Check sheet for the modelled part. Datum: model origin and axes. Units: mm. Face numbers are marked on the shaded views. A direction names the side the tool comes from. Give positions to 0.01 mm unless a question says otherwise; leave off trailing zeros. Loops run counter-clockwise (first coordinate to the right, second up) from the corner with the lowest first, then second, coordinate; pieces in that order, holes last. Notation, with made-up numbers: M 50.25,-2 L 71.25,-2 A33 ccw 71.25,30 Z; hole C 4,68 d11. An arc over 180 degrees is marked long. Write each question's results on one line, items separated by ' | '. Start each with the question number.
1. Sectioned sample at C-C on z = -3. Record the cut outline in (x, y), and give its area (3 significant figures).
2. Go/stop test with flat-tipped pins: pin 1 (7 mm diameter, centred on x = 32, y = 21.5, fed in from -Z); pin 2 (3 mm diameter, centred on y = 42.5, z = -22, fed in from +X); pin 3 (10.5 mm diameter, centred on x = -37, z = 9.5, fed in from -Y). Record where each tip stops, or that it passes through.
3. Sectioned sample at D-D on x = -39. Record the cut outline in (y, z), and give its area (3 significant figures).
4. Tool access check on the marked faces 5 and 6. Record the directions out of +Z, -Z, +X, -X, +Y, -Y that give a thin tool (end or side, any length) a straight path to the whole face; none if there is none.
5. Sectioned sample at B-B on y = 29. Record the cut outline in (x, z).
6. Material ranges on line 1 along Z through (x, y) = (0, 35); line 2 along X through (y, z) = (32, 0); line 3 along Z through (x, y) = (21, 21), recorded low to high.
7. Sectioned sample at A-A on x = 0. Record the cut outline in (y, z).
8. Draft check along Y on the marked faces 1, 2, 3 and 4. Enter one of: pulls with the +Y half, pulls with the -Y half, needs draft (parallel to the pull), parting line crosses it, or undercut.
```python
from build123d import *

# Parameters (mm, degrees)
SKETCH1_R           = 50.8
BOSS_EXTRUDE1_DEPTH = 50.8
SKETCH2_W           = 101.6
SKETCH2_H           = 101.6
CUT_EXTRUDE1_DEPTH  = 50.8
SKETCH3_W           = 101.6
SKETCH3_H           = 50.8
BOSS_EXTRUDE2_DEPTH = 25.4
SKETCH4_R           = 19.150000054
CUT_EXTRUDE2_DEPTH  = 50.8
CAVITY1_START       = -50.8
CAVITY1_DEPTH       = 101.6
SKETCH7_W           = 101.6
SKETCH7_H           = 22.400006
CUT_EXTRUDE3_DEPTH  = 0.2
SKETCH8_W           = 101.6
SKETCH8_H           = 4.242632202
CUT_EXTRUDE4_DEPTH  = 0.2
SKETCH9_W           = 101.6
SKETCH9_H           = 12.9
CUT_EXTRUDE5_DEPTH  = 0.2
SKETCH12_W          = 101.6
SKETCH12_H          = 6.55
CUT_EXTRUDE8_DEPTH  = 0.2
SKETCH13_W          = 101.6
SKETCH13_H          = 7.332348419
CUT_EXTRUDE9_DEPTH  = 0.2
FILLET3_R           = 0.2
FILLET4_R           = 0.2


with BuildPart() as part:
    # Sketch1 → Boss-Extrude1 (new body)
    with BuildSketch(Plane(origin=(0, 0, 0), x_dir=(1, 0, 0), z_dir=(0, 1, 0))):
        with Locations(Location((0, 0, 0), (0, 0, 270))):
            Circle(SKETCH1_R)
    extrude(amount=BOSS_EXTRUDE1_DEPTH)

    # Sketch2 → Cut-Extrude1 (cut)
    with BuildSketch(Plane(origin=(0, 50.8, 0), x_dir=(1, 0, 0), z_dir=(0, 1, 0))):
        with Locations((0, -50.8)):
            Rectangle(SKETCH2_W, SKETCH2_H)
    extrude(amount=-CUT_EXTRUDE1_DEPTH, mode=Mode.SUBTRACT)

    # Sketch3 → Boss-Extrude2 (add)
    with BuildSketch(Plane.XY):
        with Locations((0, 25.4)):
            Rectangle(SKETCH3_W, SKETCH3_H)
    extrude(amount=BOSS_EXTRUDE2_DEPTH)

    # Sketch4 → Cut-Extrude2 (cut)
    with BuildSketch(Plane(origin=(0, 50.8, 0), x_dir=(1, 0, 0), z_dir=(0, 1, 0))):
        with Locations(Location((0, 0, 0), (0, 0, 270))):
            Circle(SKETCH4_R)
    extrude(amount=-CUT_EXTRUDE2_DEPTH, mode=Mode.SUBTRACT)

    # Cavity1: read off the stored shape, not the designer's step
    # Cavity1 outline → Cavity1 (cut)
    with BuildSketch(Plane.YZ.offset(CAVITY1_START)):
        Polygon((19.05, 12.9), (12.7, 9.233825791), (12.7, 25.4), (0, 25.4), (0, 3.199994), (2.999994, 0.2), (25.4, 0.2), (25.4, 12.9), align=None)
    extrude(amount=CAVITY1_DEPTH, mode=Mode.SUBTRACT)

    # Sketch7 → Cut-Extrude3 (cut)
    with BuildSketch(Plane.XY.offset(0.2)):
        with Locations((0, 14.199997)):
            Rectangle(SKETCH7_W, SKETCH7_H)
    extrude(amount=-CUT_EXTRUDE3_DEPTH, mode=Mode.SUBTRACT)

    # Sketch8 → Cut-Extrude4 (cut)
    with BuildSketch(Plane(origin=(0, 1.599997, 1.599997), x_dir=(1, 0, 0), z_dir=(0, 0.7071067811865475, 0.7071067811865477))):
        with Locations((0, -0.141421356)):
            Rectangle(SKETCH8_W, SKETCH8_H)
    extrude(amount=-CUT_EXTRUDE4_DEPTH, mode=Mode.SUBTRACT)

    # Sketch9 → Cut-Extrude5 (cut)
    with BuildSketch(Plane.XZ.offset(-25.4)):
        with Locations((0, 6.45)):
            Rectangle(SKETCH9_W, SKETCH9_H)
    extrude(amount=-CUT_EXTRUDE5_DEPTH, mode=Mode.SUBTRACT)

    # Sketch12 → Cut-Extrude8 (cut)
    with BuildSketch(Plane(origin=(0, 0, 12.9), x_dir=(-1, 0, 0), z_dir=(0, 0, -1))):
        with Locations((0, 22.325)):
            Rectangle(SKETCH12_W, SKETCH12_H)
    extrude(amount=-CUT_EXTRUDE8_DEPTH, mode=Mode.SUBTRACT)

    # Sketch13 → Cut-Extrude9 (cut)
    with BuildSketch(Plane(origin=(0, -0.823363854, 1.426108029), x_dir=(-1, 0, 0), z_dir=(0, 0.4999999999999968, -0.8660254037844406))):
        with Locations((0, 19.281609733)):
            Rectangle(SKETCH13_W, SKETCH13_H)
    extrude(amount=-CUT_EXTRUDE9_DEPTH, mode=Mode.SUBTRACT)

    # Fillet3
    # the kernel refuses this fillet: 0.2 mm, written as the material it takes off along each edge
    with BuildSketch(Plane(origin=(-51.3, 19.05, 12.9), x_dir=(0, -1.0658141036380147e-12, 1.0), z_dir=(1, 0, 0))) as fillet3_piece_1:
        with BuildLine():
            CenterArc((0.373205081, 0.1), FILLET3_R, 180, 30)
            Line((0.173205081, 0.1), (0, 0))
            Line((0, 0), (0.2, 0))
        make_face()
    extrude(amount=37.646820072, mode=Mode.SUBTRACT)
    with BuildSketch(Plane(origin=(13.653179928, 19.05, 12.9), x_dir=(0, -0.4999999999991145, 0.86602540378495), z_dir=(1, 0, 0))) as fillet3_piece_2:
        with BuildLine():
            CenterArc((0.373205081, -0.1), FILLET3_R, 150, 30)
            Line((0.173205081, -0.1), (0, 0))
            Line((0, 0), (0.2, 0))
        make_face()
    extrude(amount=37.646820072, mode=Mode.SUBTRACT)

    # Fillet4
    # the kernel refuses this fillet: 0.2 mm, written as the material it takes off along each edge
    with BuildSketch(Plane(origin=(-51.3, 2.999994, 0.2), x_dir=(0, -1.4543921622385273e-11, -1.0), z_dir=(1, 0, 0))) as fillet4_piece_1:
        with BuildLine():
            CenterArc((0.341421356, -0.141421356), FILLET4_R, 135.000000001, 44.999999999)
            Line((0.141421356, -0.141421356), (0, 0))
            Line((0, 0), (0.2, 0))
        make_face()
    extrude(amount=32.651044361, mode=Mode.SUBTRACT)
    with BuildSketch(Plane(origin=(18.648955639, 2.999994, 0.2), x_dir=(0, -0.7071067811764699, -0.7071067811966253), z_dir=(1, 0, 0))) as fillet4_piece_2:
        with BuildLine():
            CenterArc((0.341421356, 0.141421356), FILLET4_R, 180, 44.999999999)
            Line((0.141421356, 0.141421356), (0, 0))
            Line((0, 0), (0.2, 0))
        make_face()
    extrude(amount=32.651044361, mode=Mode.SUBTRACT)


solid = part.part
```
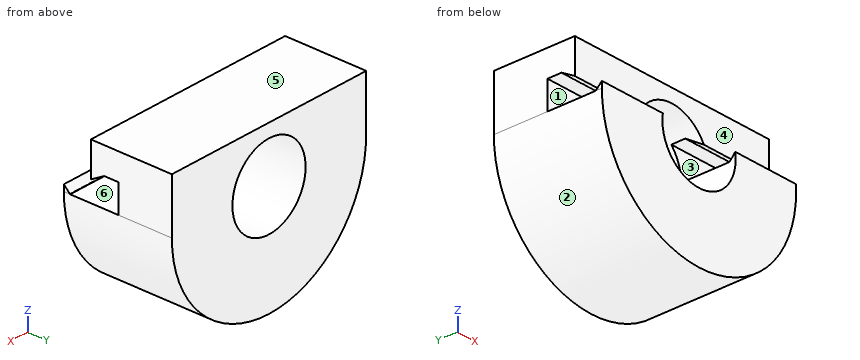
Output values:
1) outline: M -50.71,0 L -18.91,0 L -18.91,50.8 L -50.71,50.8 Z; M 18.91,0 L 50.71,0 L 50.71,50.8 L 18.91,50.8 Z | area: 3,230 mm2
2) pin 1: z = -42.05 | pin 2: x = 46.48 | pin 3: y = 12.7
3) outline: M 0,-32.55 L 50.8,-32.55 L 50.8,25.4 L 12.7,25.4 L 12.7,9.46 L 18.95,13.07 A0.2 ccw 19.05,13.1 L 25.6,13.1 L 25.6,0 L 3,0 A0.2 ccw 2.86,0.06 L 0,2.92 Z | area: 2,470 mm2
4) face 5: +Z, +X, -X, +Y, -Y | face 6: +X, -X
5) outline: M -50.8,0 A50.8 ccw 50.8,0 L 50.8,25.4 L -50.8,25.4 Z; hole C 0,0 d38.3
6) line 1: -50.8 to -19.15, 19.15 to 25.4 | line 2: -50.8 to -19.15, 19.15 to 50.8 | line 3: -46.26 to 0, 13.1 to 25.4
7) outline: M 0,-50.8 L 50.8,-50.8 L 50.8,-19.15 L 0,-19.15 Z; M 12.7,19.15 L 50.8,19.15 L 50.8,25.4 L 12.7,25.4 Z
8) face 1: undercut | face 2: needs draft | face 3: undercut | face 4: pulls with the -Y half
